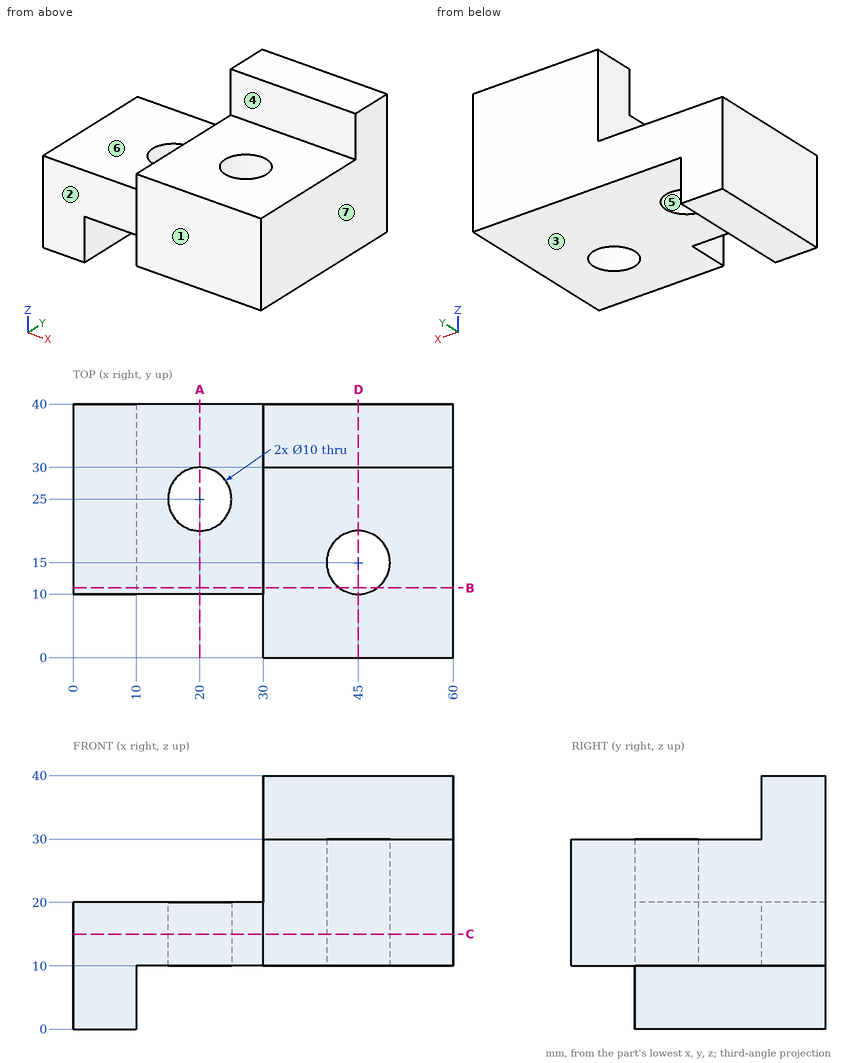
Could you check a few things on this drawing? It's one solid part, dimensions in mm from its lowest x, y, z. A direction names the side the tool comes from. Give positions to 0.01 mm unless a question says otherwise; leave off trailing zeros. Order: outer loops, then holes, each group sorted by start corner. A loop starts at its lowest first (then second) coordinate and runs counter-clockwise, first axis right, second up. Notation, with made-up numbers: (28, 3) - (72, 3) arc R24 cw to (72, 13) - close; hole circle Ø5 at (35.5, -25). An arc over 180 degrees is marked (long way). One line per question, with ' | ' between items. Start each with the question number.
Item 1: I want a section at D-D on x = 45. Write out the boundary of the cut face in (y, z), then the cut area to 3 significant figures.
Item 2: I want a section at C-C on z = 15. Write out the boundary of the cut face in (x, y).
Item 3: I'm going to push flat-ended pins straight in: pin 1 Ø6 at (y, z) = (19, 23.5) entering from -X; pin 2 Ø16 at (x, y) = (45, 15) entering from -Z; pin 3 Ø9 at (x, y) = (41, 22.5) entering from +Z; pin 4 Ø9 at (x, y) = (20, 25) entering from -Z. Where does each tip first touch, or does it pass through?
Item 4: Thinking about a two-plate mould opening in X: for the marked faces 5, 6 and 7, which applies, pulls with the +X half, pulls with the -X half, needs draft (parallel to the pull), parting line crosses it, or undercut?
Item 5: I want a section at B-B on y = 11. Write out the boundary of the cut face in (x, z), then the cut area to 3 significant figures.
Item 6: I want a section at A-A on x = 20. Write out the boundary of the cut face in (y, z), then the cut area to 3 significant figures.
Item 7: I need wall thicknesses on probe 1 along Y at (x, z) = (45, 22.5); probe 2 along Z at (x, y) = (37, 32.5); probe 3 along Z at (x, y) = (16.5, 13). Which ranges of each line are inside material? Lowest first, please. Write a range as [from, to].
Item 8: For the marked faces 1, 2, 3 and 4, which set-ups out of +Z, -Z, +X, -X, +Y, -Y let a thin tool reach every point of the face, with its end or its side?
Verdict:
1) outline: (0, 10) - (10, 10) - (10, 30) - (0, 30) - close; (20, 10) - (40, 10) - (40, 40) - (30, 40) - (30, 30) - (20, 30) - close | area: 700 mm^2
2) outline: (0, 10) - (30, 10) - (30, 0) - (60, 0) - (60, 40) - (0, 40) - close; hole circle Ø10 at (20, 25); hole circle Ø10 at (45, 15)
3) pin 1: x = 30 | pin 2: z = 10 | pin 3: z = 30 | pin 4: through
4) face 5: undercut | face 6: needs draft | face 7: pulls with the +X half
5) outline: (0, 0) - (10, 0) - (10, 10) - (42, 10) - (42, 30) - (30, 30) - (30, 20) - (0, 20) - close; (48, 10) - (60, 10) - (60, 30) - (48, 30) - close | area: 880 mm^2
6) outline: (10, 10) - (20, 10) - (20, 20) - (10, 20) - close; (30, 10) - (40, 10) - (40, 20) - (30, 20) - close | area: 200 mm^2
7) probe 1: [0, 10], [20, 40] | probe 2: [10, 40] | probe 3: [10, 20]
8) face 1: +Z, -Z, +X, -X, -Y | face 2: +Z, -Z, -X, -Y | face 3: -Z, +X, +Y, -Y | face 4: +Z, +X, -X, -Y
